Design review of the part built by this model. Coordinates are the model's own, in mm. A direction names the side the tool comes from. Give positions to 0.01 mm unless a question says otherwise; leave off trailing zeros. Loops run counter-clockwise (first coordinate to the right, second up) from the corner with the lowest first, then second, coordinate; pieces in that order, holes last.
from build123d import *

# Parameters (mm, degrees)
SKETCH_1_W      = 8.03
SKETCH_1_H      = 4.03
SKETCH_1_R      = 1.5
SKETCH_1_W_2    = 4.04
SKETCH_1_H_2    = 8.04
EXTRUDE_1_DEPTH = 4


with BuildPart() as part:
    # 草图1 → 凸台-拉伸1 (new body)
    with BuildSketch(Plane.XY):
        with BuildLine():
            Line((149, 64.5), (145, 64.5))
            Line((145, 64.5), (145, 37))
            Line((145, 37), (141, 37))
            Line((141, 37), (141, 29))
            Line((141, 29), (145, 29))
            Line((145, 29), (145, 0))
            Line((145, 0), (290, 0))
            Line((290, 0), (290, 29))
            Line((290, 29), (294, 29))
            Line((294, 29), (294, 37))
            Line((294, 37), (290, 37))
            Line((290, 37), (290, 64.5))
            Line((290, 64.5), (286, 64.5))
            Line((286, 64.5), (286, 63.15))
            Line((286, 63.15), (283.4, 63.15))
            Line((283.4, 63.15), (283.4, 64.5))
            Line((283.4, 64.5), (281.4, 64.5))
            Line((281.4, 64.5), (281.4, 67.5))
            Line((281.4, 67.5), (283.4, 67.5))
            Line((283.4, 67.5), (283.4, 68.85))
            Line((283.4, 68.85), (286, 68.85))
            Line((286, 68.85), (286, 67.5))
            Line((286, 67.5), (290, 67.5))
            Line((290, 67.5), (290, 95))
            Line((290, 95), (294, 95))
            Line((294, 95), (294, 103))
            Line((294, 103), (290, 103))
            Line((290, 103), (290, 108))
            Line((290, 108), (267.5, 108))
            Line((267.5, 108), (267.5, 67))
            ThreePointArc((267.5, 67), (264.571067812, 59.928932188), (257.5, 57))
            Line((257.5, 57), (239.5, 57))
            ThreePointArc((239.5, 57), (232.428932188, 59.928932188), (229.5, 67))
            Line((229.5, 67), (229.5, 132.57))
            Line((229.5, 132.57), (205.5, 132.57))
            Line((205.5, 132.57), (205.5, 67))
            ThreePointArc((205.5, 67), (202.571067812, 59.928932188), (195.5, 57))
            Line((195.5, 57), (177.5, 57))
            ThreePointArc((177.5, 57), (170.428932188, 59.928932188), (167.5, 67))
            Line((167.5, 67), (167.5, 108))
            Line((167.5, 108), (145, 108))
            Line((145, 108), (145, 103))
            Line((145, 103), (141, 103))
            Line((141, 103), (141, 95))
            Line((141, 95), (145, 95))
            Line((145, 95), (145, 67.5))
            Line((145, 67.5), (149, 67.5))
            Line((149, 67.5), (149, 68.85))
            Line((149, 68.85), (151.6, 68.85))
            Line((151.6, 68.85), (151.6, 67.5))
            Line((151.6, 67.5), (153.6, 67.5))
            Line((153.6, 67.5), (153.6, 64.5))
            Line((153.6, 64.5), (151.6, 64.5))
            Line((151.6, 64.5), (151.6, 63.15))
            Line((151.6, 63.15), (149, 63.15))
            Line((149, 63.15), (149, 64.5))
        make_face()
        with Locations((184.5, 4.9)):
            Rectangle(SKETCH_1_W, SKETCH_1_H, mode=Mode.SUBTRACT)
        with BuildLine():
            ThreePointArc((167.5, 36.934316811), (168.964466094, 40.469850717), (172.5, 41.934316811))
            Line((172.5, 41.934316811), (262.5, 41.934316811))
            ThreePointArc((262.5, 41.934316811), (266.035533906, 40.469850717), (267.5, 36.934316811))
            Line((267.5, 36.934316811), (267.5, 21))
            ThreePointArc((267.5, 21), (266.035533906, 17.464466094), (262.5, 16))
            Line((262.5, 16), (172.5, 16))
            ThreePointArc((172.5, 16), (168.964466094, 17.464466094), (167.5, 21))
            Line((167.5, 21), (167.5, 36.934316811))
        make_face(mode=Mode.SUBTRACT)
        with Locations((217.5, 4.9)):
            Circle(SKETCH_1_R, mode=Mode.SUBTRACT)
        with Locations((250.5, 4.9)):
            Rectangle(SKETCH_1_W, SKETCH_1_H, mode=Mode.SUBTRACT)
        with Locations((217, 69.654316811)):
            Circle(SKETCH_1_R, mode=Mode.SUBTRACT)
        with Locations((217, 95.654316811)):
            Rectangle(SKETCH_1_W_2, SKETCH_1_H_2, mode=Mode.SUBTRACT)
        with Locations((217, 121.654316811)):
            Circle(SKETCH_1_R, mode=Mode.SUBTRACT)
    extrude(amount=EXTRUDE_1_DEPTH)


solid = part.part
Q1. Tool access review of faces 1 (the face through (145, 81, 2)), 2 (the face through (143, 29, 2)), 3 (the face through (292, 37, 2)), 4 (the face through (250, 6.915, 2)), 5 (the face through (167.5, 87, 2)): name each direction out of +Z, -Z, +X, -X, +Y, -Y from which nothing blocks a thin tool from reaching the whole face with its end or side.
Results:
face 1: +Z, -Z, -X
face 2: +Z, -Z, -X, -Y
face 3: +Z, -Z, +X
face 4: +Z, -Z
face 5: +Z, -Z, +Y
Q2. Insertion check: pin 1 (2 mm diameter, centred on x = 288, z = 1.5, fed in from +Y); pin 2 (1.5 mm diameter, centred on y = 64, z = 3, fed in from -X); pin 3 (2 mm diameter, centred on x = 142, z = 1.5, fed in from +Y). Each pin has a flat end and moves straight along its axis. Give the tip position at first contact, or say it passes through.
Results:
pin 1: stops at y = 108
pin 2: stops at x = 145
pin 3: stops at y = 103
Q3. Draft analysis for pull direction Y (two halves, no side actions). For faces 6 (the face through (170.51, 59.85, 1.97)), 7 (the face through (290, 105, 2)), 8 (the face through (188.515, 5, 2)), state which applies: pulls with the +Y half, pulls with the -Y half, needs draft (parallel to the pull), parting line crosses it, or undercut.
Results:
face 6: pulls with the +Y half
face 7: needs draft
face 8: undercut
Q4. Take a section at A-A (x = 243.5). Give the boundary of the cut face in (y, z).
Results:
outline: (0, 0) - (16, 0) - (16, 4) - (0, 4) - close; (41.93, 0) - (57, 0) - (57, 4) - (41.93, 4) - close
Q5. Wall thickness on line 1 (X direction, y = 76, z = 1.1); line 2 (X direction, y = 100, z = 0.8); line 3 (X direction, y = 99, z = 2.1): over which ranges is each line inside the solid? List them lowest first.
Results:
line 1: x = 145 to 167.5, 205.5 to 229.5, 267.5 to 290
line 2: x = 141 to 167.5, 205.5 to 229.5, 267.5 to 294
line 3: x = 141 to 167.5, 205.5 to 214.98, 219.02 to 229.5, 267.5 to 294
Q6. Take a section at C-C (y = 113.5). Give the boundary of the cut face in (x, z).
Results:
outline: (205.5, 0) - (229.5, 0) - (229.5, 4) - (205.5, 4) - close
Q7. Take a section at D-D (x = 273.5). Give the boundary of the cut face in (y, z), plus the area to 3 significant figures.
Results:
outline: (0, 0) - (108, 0) - (108, 4) - (0, 4) - close
area: 432 mm2
Q8. Take a section at B-B (y = 40). Give the boundary of the cut face in (x, z), plus the area to 3 significant figures.
Results:
outline: (145, 0) - (168.55, 0) - (168.55, 4) - (145, 4) - close; (266.45, 0) - (290, 0) - (290, 4) - (266.45, 4) - close
area: 188 mm2
